from build123d import *

# Parameters (mm, degrees)
F1_DEPTH = 20
F2_R     = 5
F3_R     = 5
F4_ANGLE = 90


with BuildPart() as f1:
    # F0 (on Front) → F1 (new body)
    with BuildSketch(Plane.XZ):
        with BuildLine():
            Line((32, 39), (5, 39))
            ThreePointArc((5, 39), (1.4644660941, 37.5355339059), (0, 34))
            Line((0, 34), (0, 29))
            Line((0, 29), (20, 29))
            ThreePointArc((20, 29), (23.5355339059, 27.5355339059), (25, 24))
            Line((25, 24), (25, 15))
            ThreePointArc((25, 15), (23.5355339059, 11.4644660941), (20, 10))
            Line((20, 10), (0, 10))
            Line((0, 10), (0, 0))
            Line((0, 0), (72, 0))
            ThreePointArc((72, 0), (75.5355339059, 1.4644660941), (77, 5))
            Line((77, 5), (77, 20))
            Line((77, 20), (67, 20))
            Line((67, 20), (67, 17))
            ThreePointArc((67, 17), (65.5355339059, 13.4644660941), (62, 12))
            Line((62, 12), (42, 12))
            ThreePointArc((42, 12), (38.4644660941, 13.4644660941), (37, 17))
            Line((37, 17), (37, 34))
            ThreePointArc((37, 34), (35.5355339059, 37.5355339059), (32, 39))
        make_face()
    extrude(amount=F1_DEPTH)

    # F2
    f2_edges = [f1.edges().sort_by_distance(p)[0] for p in [
        (67, -10, 20),
    ]]
    fillet(f2_edges, radius=F2_R)

    # F3
    f3_edges = [f1.edges().sort_by_distance(p)[0] for p in [
        (77, -10, 20),
    ]]
    fillet(f3_edges, radius=F3_R)


with BuildPart() as f1_1:
    # F4: moved
    add(f1.part.rotate(Axis((36, 0, 0), (-1, 0, 0)), F4_ANGLE))


solid = f1_1.part
For this review, take the finished solid that the model builds, in its own axes (mm). A direction names the side the tool comes from. Give positions to 0.01 mm unless a question says otherwise; leave off trailing zeros. Order: outer loops, then holes, each group sorted by start corner. A loop starts at its lowest first (then second) coordinate and runs counter-clockwise, first axis right, second up. Notation, with made-up numbers: M -33.5,37.25 L -12.5,37.25 A37 ccw -12.5,74.25 Z; hole C 43.25,68 d5. An arc over 180 degrees is marked long. Answer in a Markdown table with one row per item. Add a question column.
(1) For pin 1 (5 mm diameter, centred on y = 24.5, z = 8, fed in from +X); pin 2 (10 mm diameter, centred on x = 55, z = 16, fed in from +Y); pin 3 (7 mm diameter, centred on y = 19.5, z = 12, fed in from -X), all flat-tipped, find the tip position at first contact; note any pin that passes through.
(2) Wall thickness on probe 1 along Y at (x, z) = (8, 4); probe 2 along Y at (x, z) = (46, 4.5); probe 3 along X at (y, z) = (30, 6): over which ranges is each line inside the solid? List them lowest first. Write a range as [from, to].
(3) Consider section B-B on x = 65. State the section outline as (y, z) points, and give its area (3 significant figures).
(4) Mouldability with a two-part tool opening along X and no side actions: class faces 4 (the face through (25, 20, 10)), 5 (the face through (75, 19, 10)), 6 (the face through (35, 0, 10)), 7 (the face through (37, 25, 10)) as +X half, -X half, draft (parallel to the pull), parting line (faces both ways), or undercut.
(5) Consider section A-A on x = 7. State the section outline as (y, z) points, and give its area (3 significant figures).
(6) For faces 1 (the face through (10, 10, 10)), 2 (the face through (65, 13, 10)), 3 (the face through (75, 1, 10)), list the 3-axis set-ups (+Z, -Z, +X, -X, +Y, -Y) from which the entire face can be reached by the end or side of a thin tool; tool diameter is ignored.
Evaluation:
| question | item | result |
|---|---|---|
| 1 | pin 1 | stops at x = 37 |
| 1 | pin 2 | stops at y = 12 |
| 1 | pin 3 | stops at x = 25 |
| 2 | probe 1 | y = [0, 10], [29, 39] |
| 2 | probe 2 | y = [0, 12] |
| 2 | probe 3 | x = [0, 37] |
| 3 | outline | M 0,0 L 13,0 L 13,20 L 0,20 Z |
| 3 | area | 260 mm^2 |
| 4 | face 4 | -X half |
| 4 | face 5 | +X half |
| 4 | face 6 | draft |
| 4 | face 7 | undercut |
| 5 | outline | M 0,0 L 10,0 L 10,20 L 0,20 Z; M 29,0 L 39,0 L 39,20 L 29,20 Z |
| 5 | area | 400 mm^2 |
| 6 | face 1 | +Z, -Z, -X |
| 6 | face 2 | +Z, -Z, +Y |
| 6 | face 3 | +Z, -Z, +X, -Y |
